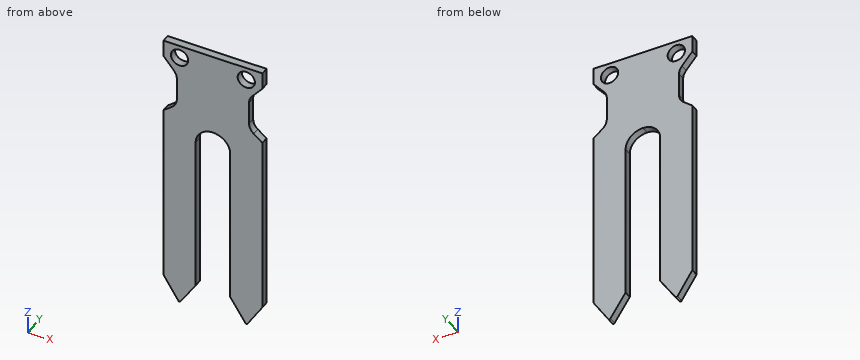
```python
from build123d import *

# Parameters (mm, degrees)
F0_R     = 1.75
F1_DEPTH = 1.53
F2_R     = 0.25
F3_R     = 2.5


with BuildPart() as f1:
    # F0 (on Front) → F1 (new body)
    with BuildSketch(Plane.XZ):
        with BuildLine():
            Line((10, 0), (0, 0))
            Line((0, 0), (-10, 0))
            Line((-10, 0), (-10, -3.44))
            Line((-10, -3.44), (-7.303071, -6.615652))
            Line((-7.303071, -6.615652), (-7.303071, -13.405652))
            Line((-7.303071, -13.405652), (-10, -15.541108))
            Line((-10, -15.541108), (-10, -52.352146))
            Line((-10, -52.352146), (-6.78713, -57.41944))
            Line((-6.78713, -57.41944), (-3.5, -52.4))
            Line((-3.5, -52.4), (-3.5, -20.4))
            ThreePointArc((-3.5, -20.4), (-2.474874, -17.925126), (0, -16.9))
            ThreePointArc((0, -16.9), (2.474874, -17.925126), (3.5, -20.4))
            Line((3.5, -20.4), (3.5, -52.4))
            Line((3.5, -52.4), (6.78713, -57.41944))
            Line((6.78713, -57.41944), (10, -52.352146))
            Line((10, -52.352146), (10, -15.541108))
            Line((10, -15.541108), (7.303071, -13.405652))
            Line((7.303071, -13.405652), (7.303071, -6.615652))
            Line((7.303071, -6.615652), (10, -3.44))
            Line((10, -3.44), (10, 0))
        make_face()
        with Locations((-6.75, -2.616455)):
            Circle(F0_R, mode=Mode.SUBTRACT)
        with Locations((6.75, -2.616455)):
            Circle(F0_R, mode=Mode.SUBTRACT)
    extrude(amount=F1_DEPTH)

    # F2
    f2_edges = [f1.edges().sort_by_distance(p)[0] for p in [
        (-6.78713, -0.765, -57.41944),
        (6.78713, -0.765, -57.41944),
    ]]
    fillet(f2_edges, radius=F2_R)

    # F3
    f3_edges = [f1.edges().sort_by_distance(p)[0] for p in [
        (-7.303071, -0.765, -13.405652),
        (-7.303071, -0.765, -6.615652),
        (7.303071, -0.765, -6.615652),
        (7.303071, -0.765, -13.405652),
    ]]
    fillet(f3_edges, radius=F3_R)


solid = f1.part
```
Verification items for the finished model (mm, model axes). Give positions to 0.01 mm unless a question says otherwise; leave off trailing zeros. Order: outer loops, then holes, each group sorted by start corner. A loop starts at its lowest first (then second) coordinate and runs counter-clockwise, first axis right, second up. Notation, with made-up numbers: (45, 50) -> (94, 50) arc R4 ccw to (94, 55) -> close; hole circle Ø3 at (70.25, -35). An arc over 180 degrees is marked (long way). Use a Markdown table: item, result.
1) Depth check by flat-ended pin: pin 1 Ø1 at (x, z) = (-7.5, -47) entering from +Y. Enter the tip coordinate at first touch or a pass-through.
Results:
| item | result |
|---|---|
| pin 1 | y = 0 |
2) Section check D-D, the plane x = -2.75. Record the boundary of the cut face in (y, z).
Results:
| item | result |
|---|---|
| outline | (-1.53, -18.23) -> (0, -18.23) -> (0, 0) -> (-1.53, 0) -> close |
3) Section check B-B, the plane y = -0.6. Record the boundary of the cut face in (x, z), then the cut area to 3 significant figures.
Results:
| item | result |
|---|---|
| outline | (-10, -52.35) -> (-6.99, -57.09) arc R0.25 ccw to (-6.57, -57.09) -> (-3.5, -52.4) -> (-3.5, -20.4) arc R3.5 cw to (0, -16.9) arc R3.5 cw to (3.5, -20.4) -> (3.5, -52.4) -> (6.57, -57.09) arc R0.25 ccw to (6.99, -57.09) -> (10, -52.35) -> (10, -15.54) -> (8.25, -14.16) arc R2.5 cw to (7.3, -12.2) -> (7.3, -7.53) arc R2.5 cw to (7.9, -5.92) -> (10, -3.44) -> (10, 0) -> (-10, 0) -> (-10, -3.44) -> (-7.9, -5.92) arc R2.5 cw to (-7.3, -7.53) -> (-7.3, -12.2) arc R2.5 cw to (-8.25, -14.16) -> (-10, -15.54) -> close; hole circle Ø3.5 at (-6.75, -2.62); hole circle Ø3.5 at (6.75, -2.62) |
| area | 768 mm² |
4) Section check C-C, the plane z = -11.5. Record the boundary of the cut face in (x, y).
Results:
| item | result |
|---|---|
| outline | (-7.3, -1.53) -> (7.3, -1.53) -> (7.3, 0) -> (-7.3, 0) -> close |
5) Section check A-A, the plane z = -42.5. Record the boundary of the cut face in (x, y).
Results:
| item | result |
|---|---|
| outline | (-10, -1.53) -> (-3.5, -1.53) -> (-3.5, 0) -> (-10, 0) -> close; (3.5, -1.53) -> (10, -1.53) -> (10, 0) -> (3.5, 0) -> close |
6) Material ranges on probe 1 along X at (y, z) = (-1.15, -39.5); probe 2 along Z at (x, y) = (6.75, -0.8); probe 3 along X at (y, z) = (-0.4, -53), recorded low to high.
Results:
| item | result |
|---|---|
| probe 1 | -10 to -3.5, 3.5 to 10 |
| probe 2 | -57.21 to -4.37, -0.87 to 0 |
| probe 3 | -9.59 to -3.89, 3.89 to 9.59 |
